The drawing under review shows one solid part. Ordinate dimensions are in mm from its lowest x, y, z. Coordinates: 2 decimals unless noted, no trailing zeros. Write each loop counter-clockwise with the first axis right and the second up, starting at its lowest first coordinate (ties: lowest second). Pieces come first, ordered by that corner, then holes. Notation, with made-up numbers: M -30,42.5 L -9,42.5 A8 ccw -9,51.5 Z; hole C -20.75,-18.5 d6. An arc over 180 degrees is marked long. Write item = value, one per line.
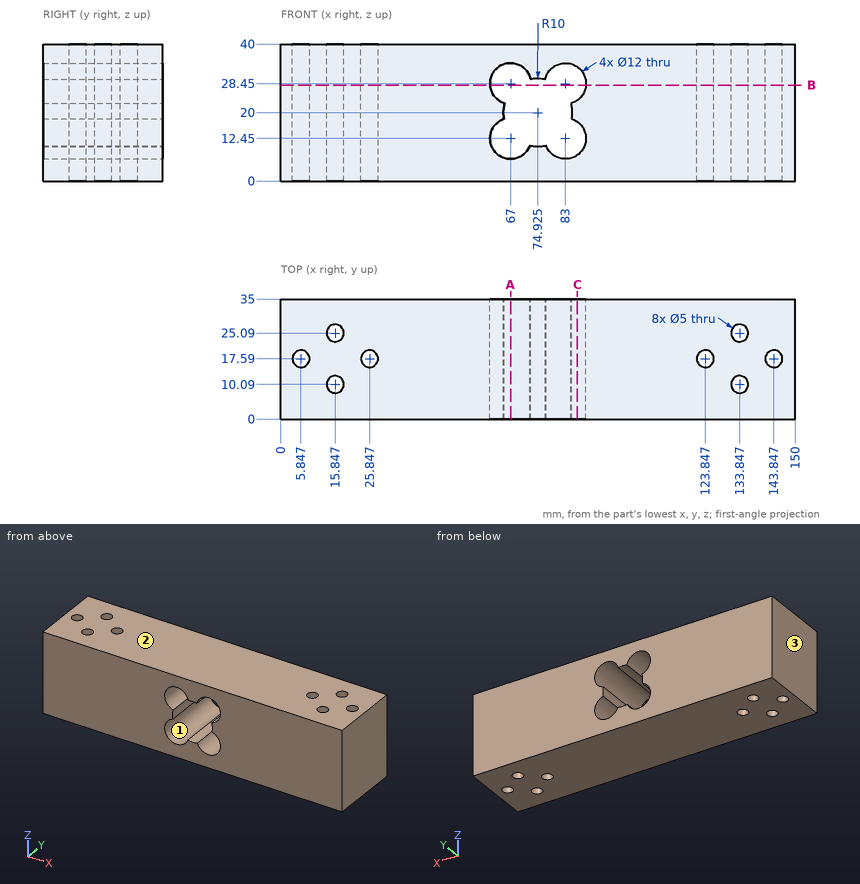
Q1. Consider section A-A, the plane x = 67. State the section outline as (y, z) points.
Check result:
outline = M 0,0 L 35,0 L 35,6.45 L 0,6.45 Z; M 0,34.45 L 35,34.45 L 35,40 L 0,40 Z
Q2. For P1, Ø3, axis at x = 5.85, y = 17.59, coming from the +Z side, flat-tipped, find the tip position at first contact; note if it passes through.
Check result:
P1 = through
Q3. Consider section C-C, the plane x = 86.5. State the section outline as (y, z) points, and give its area (3 significant figures).
Check result:
outline = M 0,0 L 35,0 L 35,7.58 L 0,7.58 Z; M 0,17.32 L 35,17.32 L 35,23.58 L 0,23.58 Z; M 0,33.32 L 35,33.32 L 35,40 L 0,40 Z
area = 718 mm²
Q4. Consider section B-B, the plane z = 28. State how many separate pieces and enclosed holes the cut face has, and give its area (3 significant figures).
Check result:
separate_pieces = 2
enclosed_holes = 8
area = 4,110 mm²
Q5. The part is to be moulded in two halves that separate along X. For the marked faces 1, 2 and 3, say which applies: +X half, -X half, draft (parallel to the pull), parting line (faces both ways), or undercut.
Check result:
face_1 = undercut
face_2 = draft
face_3 = -X half
Q6. Wall thickness on line 1 (Y direction, x = 26, z = 18) (1 decimal); line 2 (X direction, y = 17, z = 28.5); line 3 (X direction, y = 26.5, z = 19.5): over which ranges is each line inside the solid? List them lowest first.
Check result:
line_1 = 0 to 15.1, 20.1 to 35
line_2 = 0 to 3.42, 8.28 to 23.42, 28.28 to 61, 89 to 121.42, 126.28 to 141.42, 146.28 to 150
line_3 = 0 to 13.78, 17.91 to 64.94, 84.91 to 131.78, 135.91 to 150
